The drawing under review shows one solid part. Ordinate dimensions are in mm from its lowest x, y, z. A direction names the side the tool comes from. Round coordinates to 2 decimals unless told otherwise and drop trailing zeros. Loops run counter-clockwise (first coordinate to the right, second up) from the corner with the lowest first, then second, coordinate; pieces in that order, holes last. Notation, with made-up numbers: (11, 24) -> (46, 24) arc R16 ccw to (46, 28) -> close; hole circle Ø6 at (65, 55). An arc over 180 degrees is marked (long way). Answer as CSV lines item,"result". Start each with the question number.
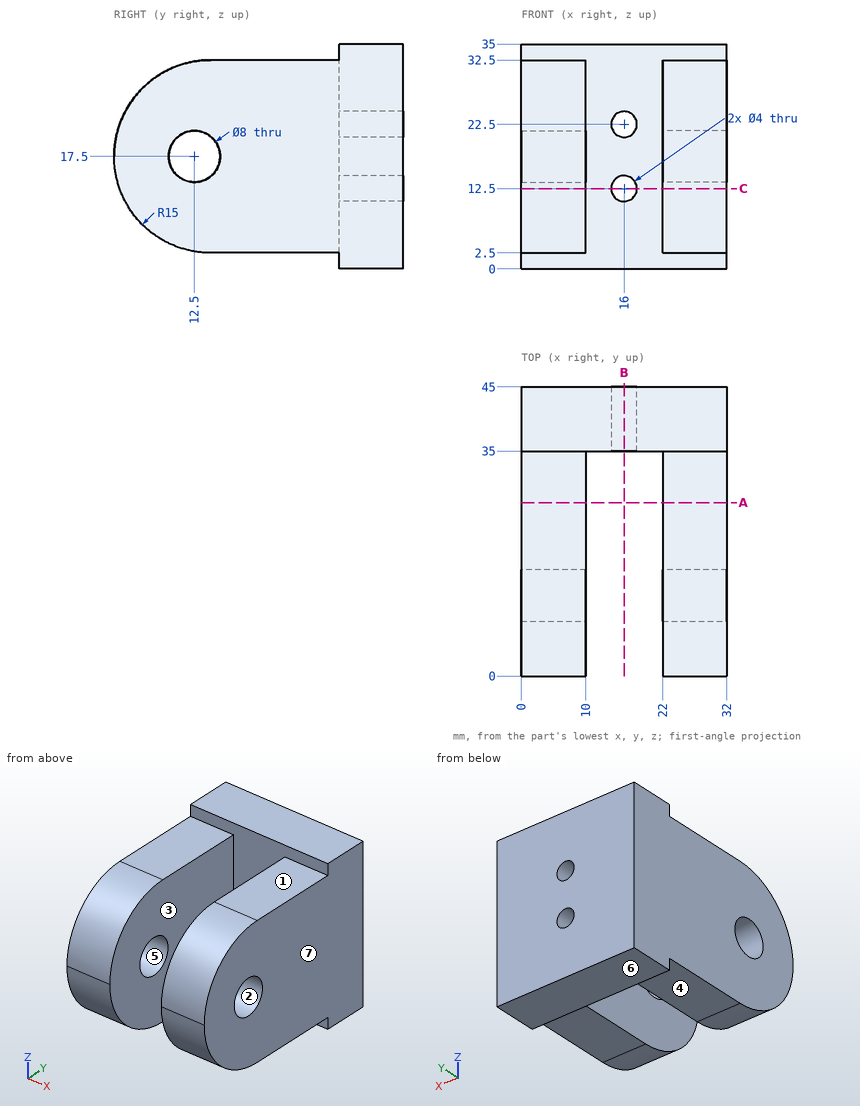
Q1. Add section A-A, the plane y = 27. Give the boundary of the cut face in (x, z).
Q2. Add section B-B, the plane x = 16. Give the boundary of the cut face in (y, z), and give its area (3 significant figures).
Q3. Mouldability with a two-part tool opening along Z and no side actions: class the marked faces 5, 6 and 7 as pulls with the +Z half, pulls with the -Z half, needs draft (parallel to the pull), parting line crosses it, or undercut.
Q4. To check wall thickness, follow probe 1 along Z at (x, y) = (16, 41); probe 2 along X at (y, z) = (32, 27); probe 3 along Y at (x, z) = (18.5, 9). State the ranges of each line that lie inside material, in increasing order. Write a range as from..to.
Q5. Add section C-C, the plane z = 12.5. Give the boundary of the cut face in (x, y).
Q6. For pin 1 Ø10 at (x, y) = (16.5, 6.5) entering from -Z; pin 2 Ø3 at (x, y) = (5.5, 28.5) entering from -Z; pin 3 Ø11 at (x, y) = (5.5, 20) entering from +Z; pin 4 Ø10 at (x, z) = (23.5, 9) entering from -Y, all flat-tipped, find the tip position at first contact; note any pin that passes through.
Q7. Machinability: for the marked faces 1, 2, 3 and 4, which of the approach directions +Z, -Z, +X, -X, +Y, -Y give a long, thin tool a straight path to every point of the face, cutting with its end or side? Answer none if there is none.
Worked answers:
1,outline,"(0, 2.5) -> (10, 2.5) -> (10, 32.5) -> (0, 32.5) -> close; (22, 2.5) -> (32, 2.5) -> (32, 32.5) -> (22, 32.5) -> close"
2,outline,"(35, 0) -> (45, 0) -> (45, 10.5) -> (35, 10.5) -> close; (35, 14.5) -> (45, 14.5) -> (45, 20.5) -> (35, 20.5) -> close; (35, 24.5) -> (45, 24.5) -> (45, 35) -> (35, 35) -> close"
2,area,"270 mm^2"
3,face 5,"undercut"
3,face 6,"pulls with the -Z half"
3,face 7,"needs draft"
4,probe 1,"z = 0..10.5, 14.5..20.5, 24.5..35"
4,probe 2,"x = 0..10, 22..32"
4,probe 3,"y = 35..45"
5,outline,"(0, 0.86) -> (10, 0.86) -> (10, 35) -> (14, 35) -> (14, 45) -> (0, 45) -> close; (18, 35) -> (22, 35) -> (22, 0.86) -> (32, 0.86) -> (32, 45) -> (18, 45) -> close"
6,pin 1,"passes through"
6,pin 2,"stops at z = 2.5"
6,pin 3,"stops at z = 32.5"
6,pin 4,"stops at y = 0.41"
7,face 1,"+Z, +X, -X, -Y"
7,face 2,"+X, -X"
7,face 3,"+Z, -Z, -Y"
7,face 4,"-Z, +X, -X, -Y"
